Here's how the part is built. I have some questions about the finished solid (model axes, mm). Face numbers are marked on the shaded views. A direction names the side the tool comes from. Round coordinates to 2 decimals unless told otherwise and drop trailing zeros. Loops run counter-clockwise (first coordinate to the right, second up) from the corner with the lowest first, then second, coordinate; pieces in that order, holes last. Notation, with made-up numbers: M 15,-6.75 L 66,-6.75 A15 ccw 66,19.25 Z; hole C 3.25,-16.75 d10. An arc over 180 degrees is marked long. Use a Markdown table: item, result.
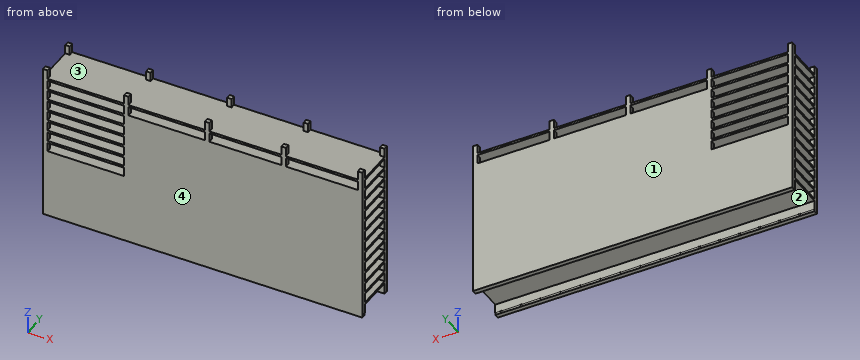
from build123d import *

# Parameters (mm, degrees)
F0_W     = 360.68
F0_H     = 50.8
F1_DEPTH = 177.8
F2_W     = 40.64
F2_H     = 10.16
F2_H_2   = 7.62
F2_H_3   = 2.54
F3_DEPTH = 360.681
F4_W     = 86.36
F4_H     = 10.16
F4_W_2   = 81.28
F5_DEPTH = 50.801
F7_DEPTH = 360.681


with BuildPart() as f1:
    # F0 (on Top) → F1 (new body)
    with BuildSketch(Plane.XY):
        with Locations((-123.650887, 16.643145)):
            Rectangle(F0_W, F0_H)
    extrude(amount=F1_DEPTH)

    # F2 (on face) → F3 (cut, through all)
    with BuildSketch(Plane(origin=(-303.990887, 0, 0), x_dir=(0, -1, 0), z_dir=(-1, 0, 0))):
        with Locations((-16.643145, 7.62)):
            Rectangle(F2_W, F2_H)
        with Locations((-16.643145, 20.32)):
            Rectangle(F2_W, F2_H)
        with Locations((-16.643145, 33.02)):
            Rectangle(F2_W, F2_H)
        with Locations((-16.643145, 45.72)):
            Rectangle(F2_W, F2_H)
        with Locations((-16.643145, 57.15)):
            Rectangle(F2_W, F2_H_2)
        with Locations((-16.643145, 62.23)):
            Rectangle(F2_W, F2_H_3)
        with Locations((-16.643145, 71.12)):
            Rectangle(F2_W, F2_H)
        with Locations((-16.643145, 83.82)):
            Rectangle(F2_W, F2_H)
        with Locations((-16.643145, 96.52)):
            Rectangle(F2_W, F2_H)
        with Locations((-16.643145, 109.22)):
            Rectangle(F2_W, F2_H)
        with Locations((-16.643145, 121.92)):
            Rectangle(F2_W, F2_H)
        with Locations((-16.643145, 134.62)):
            Rectangle(F2_W, F2_H)
        with Locations((-16.643145, 147.32)):
            Rectangle(F2_W, F2_H)
        with Locations((-16.643145, 160.02)):
            Rectangle(F2_W, F2_H)
        with Locations((-16.643145, 172.72)):
            Rectangle(F2_W, F2_H)
    extrude(amount=-F3_DEPTH, mode=Mode.SUBTRACT)

    # F4 (on face) → F5 (cut, through all)
    with BuildSketch(Plane.XZ.offset(8.756855)):
        with Locations((-255.730887, 172.72)):
            Rectangle(F4_W, F4_H)
        with Locations((-164.290887, 172.72)):
            Rectangle(F4_W, F4_H)
        with Locations((-164.290887, 160.02)):
            Rectangle(F4_W, F4_H)
        with Locations((-75.390887, 172.72)):
            Rectangle(F4_W_2, F4_H)
        with Locations((-75.390887, 160.02)):
            Rectangle(F4_W_2, F4_H)
        with Locations((10.969113, 172.72)):
            Rectangle(F4_W_2, F4_H)
        with Locations((10.969113, 160.02)):
            Rectangle(F4_W_2, F4_H)
        with Locations((-255.730887, 160.02)):
            Rectangle(F4_W, F4_H)
        with Locations((-255.730887, 147.32)):
            Rectangle(F4_W, F4_H)
        with Locations((-255.730887, 134.62)):
            Rectangle(F4_W, F4_H)
        with Locations((-255.730887, 121.92)):
            Rectangle(F4_W, F4_H)
        with Locations((-255.730887, 109.22)):
            Rectangle(F4_W, F4_H)
        with Locations((-255.730887, 96.52)):
            Rectangle(F4_W, F4_H)
        with Locations((-255.730887, 83.82)):
            Rectangle(F4_W, F4_H)
    extrude(amount=-F5_DEPTH, mode=Mode.SUBTRACT)

    # F6 (on face) → F7 (cut, through all)
    with BuildSketch(Plane(origin=(-303.990887, 0, 0), x_dir=(0, -1, 0), z_dir=(-1, 0, 0))):
        Polygon((3.676855, 2.54), (-36.963145, 2.54), (-36.963145, 0), (3.705695, 0), (3.705695, 2.54), align=None)
    extrude(amount=-F7_DEPTH, mode=Mode.SUBTRACT)


solid = f1.part
1. For pin 1 Ø2 at (x, y) = (-228.5, 12) entering from +Z; pin 2 Ø12 at (x, y) = (-235.5, 19) entering from -Z, each with a flat end and sliding along its axis, tell me the tip position at first contact or that it passes through.
Answer sheet:
| item | result |
|---|---|
| pin 1 | z = 167.64 |
| pin 2 | z = 12.7 |
2. We'd pull the mould along X, two halves only. Please class the marked faces 3 and 4: +X half, -X half, draft (parallel to the pull), parting line (faces both ways), or undercut.
Answer sheet:
| item | result |
|---|---|
| face 3 | undercut |
| face 4 | draft |
3. I need wall thicknesses on probe 1 along Y at (x, z) = (-92, 46.5). Which ranges of the line are inside material? Lowest first, please. Write a range as from..to.
Answer sheet:
| item | result |
|---|---|
| probe 1 | -8.76..-3.68, 36.96..42.04 |
4. Imagine slicing it at A-A, the plane z = 31.5. Write out the boundary of the cut face in (x, y).
Answer sheet:
| item | result |
|---|---|
| outline | M -303.99,-8.76 L 56.69,-8.76 L 56.69,-3.68 L -303.99,-3.68 Z; M -303.99,36.96 L 56.69,36.96 L 56.69,42.04 L -303.99,42.04 Z |
5. Which directions (+Z, -Z, +X, -X, +Y, -Y) give clear straight access to the entire face, cutting with the end or side of a thin tool? Please do the marked faces 1 and 2.
Answer sheet:
| item | result |
|---|---|
| face 1 | +Z, -Z, +X, -X, +Y |
| face 2 | -Z, +X, -X |
6. Imagine slicing it at B-B, the plane x = -235. State how many separate pieces and enclosed holes the cut face has, then the cut area to 3 significant figures.
Answer sheet:
| item | result |
|---|---|
| separate pieces | 8 |
| enclosed holes | 5 |
| area | 2,320 mm2 |
